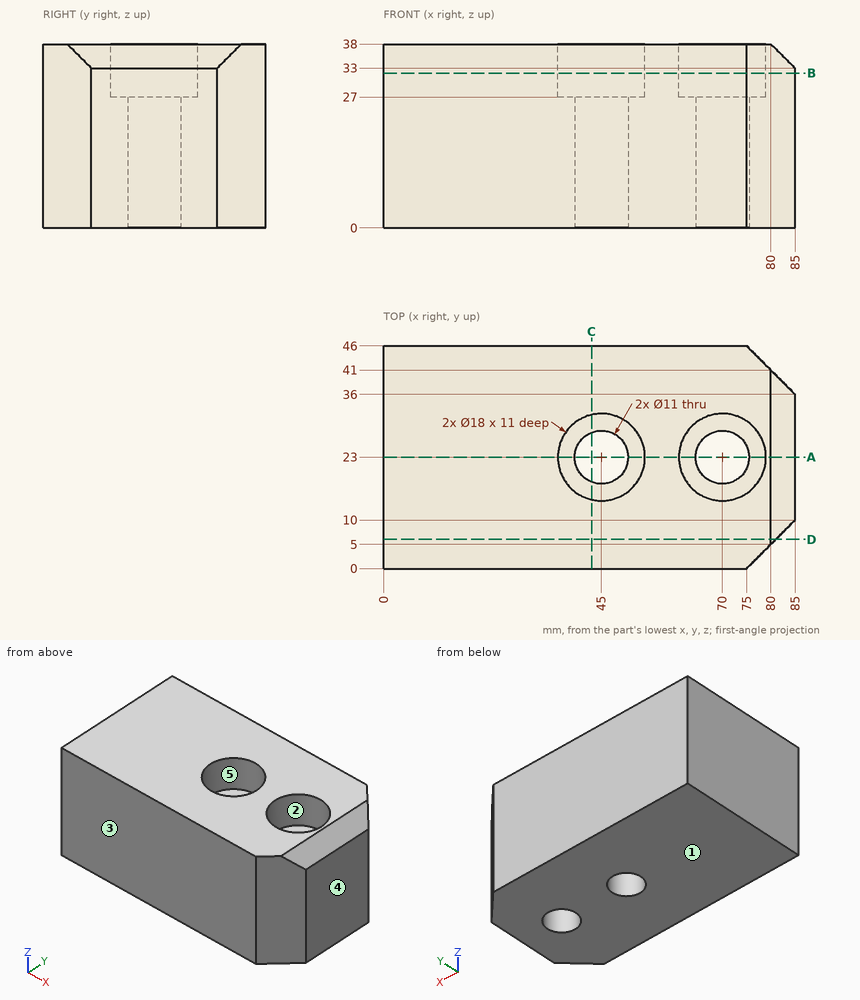
Here's the drawing with two shaded views (mm, measured from the low corner). I have some questions. A direction names the side the tool comes from. Give positions to 0.01 mm unless a question says otherwise; leave off trailing zeros. Loops run counter-clockwise (first coordinate to the right, second up) from the corner with the lowest first, then second, coordinate; pieces in that order, holes last. Notation, with made-up numbers: (6.5, 46.5) -> (50.5, 46.5) arc R23 cw to (50.5, 61.5) -> close; hole circle Ø1 at (58, 12). An arc over 180 degrees is marked (long way). One line per item, written item: value.
Q1. Suppose I cut it at D-D on y = 6. Please give me the cut outline in (x, z).
Answers follow:
outline: (0, 0) -> (81, 0) -> (81, 37) -> (80, 38) -> (0, 38) -> close
Q2. Suppose I cut it at C-C on x = 43. Please give me the cut outline in (y, z), then the cut area to 3 significant figures.
Answers follow:
outline: (0, 0) -> (17.88, 0) -> (17.88, 27) -> (14.23, 27) -> (14.23, 38) -> (0, 38) -> close; (28.12, 0) -> (46, 0) -> (46, 38) -> (31.77, 38) -> (31.77, 27) -> (28.12, 27) -> close
area: 1,280 mm^2
Q3. We'd pull the mould along Y, two halves only. Please class the marked faces 1, 2 and 3: pulls with the +Y half, pulls with the -Y half, needs draft (parallel to the pull), parting line crosses it, or undercut.
Answers follow:
face 1: needs draft
face 2: undercut
face 3: pulls with the -Y half
Q4. Suppose I cut it at A-A on y = 23. Please give me the cut outline in (x, z), then the cut area to 3 significant figures.
Answers follow:
outline: (0, 0) -> (39.5, 0) -> (39.5, 27) -> (36, 27) -> (36, 38) -> (0, 38) -> close; (50.5, 0) -> (64.5, 0) -> (64.5, 27) -> (61, 27) -> (61, 38) -> (54, 38) -> (54, 27) -> (50.5, 27) -> close; (75.5, 0) -> (85, 0) -> (85, 33) -> (80, 38) -> (79, 38) -> (79, 27) -> (75.5, 27) -> close
area: 2,230 mm^2
Q5. I'm going to push flat-ended pins straight in: pin 1 Ø20 at (x, y) = (45.5, 27.5) entering from +Z; pin 2 Ø17.5 at (x, y) = (45, 23) entering from +Z. Where does each tip first touch, or does it pass through?
Answers follow:
pin 1: z = 38
pin 2: z = 27
Q6. If I drill on line 1 along Y through (x, z) = (45, 22); line 2 along Y through (x, z) = (45, 31.25); line 3 along X through (y, z) = (17, 36), over which ranges is the centre line in solid material (lowest first)?
Answers follow:
line 1: 0 to 17.5, 28.5 to 46
line 2: 0 to 14, 32 to 46
line 3: 0 to 38.29, 51.71 to 63.29, 76.71 to 82
Q7. Suppose I cut it at B-B on z = 32. Please give me the cut outline in (x, y), then the cut area to 3 significant figures.
Answers follow:
outline: (0, 0) -> (75, 0) -> (85, 10) -> (85, 36) -> (75, 46) -> (0, 46) -> close; hole circle Ø18 at (45, 23); hole circle Ø18 at (70, 23)
area: 3,300 mm^2
Q8. On a 3-axis mill with a long thin cutter (end or side, diameter ignored), from which of +Z, -Z, +X, -X, +Y, -Y can I reach the whole of each face in a straight line? I mean the marked faces 4 and 5. Say none if no direction works.
Answers follow:
face 4: +Z, -Z, +X, +Y, -Y
face 5: +Z
